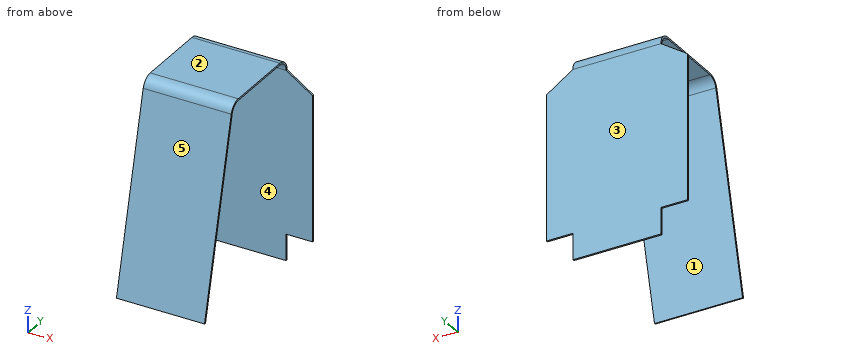
```python
from build123d import *

# Parameters (mm, degrees)
EXTRUDE_1_DEPTH      = 1.25
EXTRUDE_1_DEPTH_BACK = 1.25
SKETCH_2_W           = 4.631165465
SKETCH_2_H           = 0.05
EXTRUDE_1_2_DEPTH    = 0.75
CHAMFER_1_SIZE2      = 0.5
CHAMFER_1_SIZE       = 0.75
CHAMFER_2_SIZE2      = 0.5
CHAMFER_2_SIZE       = 0.75


with BuildPart() as part:
    # Эскиз1 → Extrude 1 (new, two sides: drawn at the far end of the back side and taken through both)
    with BuildSketch(Plane(origin=(0, 0, 0), x_dir=(0, 0, -1), z_dir=(1, 0, 0)).offset(-EXTRUDE_1_DEPTH_BACK)):
        with BuildLine():
            Line((0, 0), (-5.38, 0))
            ThreePointArc((-5.38, 0), (-5.592132034, -0.087867966), (-5.68, -0.3))
            Line((-5.68, -0.3), (-5.68, -2.314556047))
            ThreePointArc((-5.68, -2.314556047), (-5.615998777, -2.499770997), (-5.451302817, -2.60595939))
            Line((-5.451302817, -2.60595939), (-0.162763373, -3.9))
            Line((-0.162763373, -3.9), (-0.174647176, -3.948567224))
            Line((-0.174647176, -3.948567224), (-5.46318662, -2.654526614))
            ThreePointArc((-5.46318662, -2.654526614), (-5.655331906, -2.530640155), (-5.73, -2.314556047))
            Line((-5.73, -2.314556047), (-5.73, -0.3))
            ThreePointArc((-5.73, -0.3), (-5.627487373, -0.052512627), (-5.38, 0.05))
            Line((-5.38, 0.05), (0, 0.05))
            Line((0, 0.05), (0, 0))
        make_face()
    extrude(amount=EXTRUDE_1_DEPTH + EXTRUDE_1_DEPTH_BACK)

    # Эскиз2 → Extrude 1 2 (add)
    with BuildSketch(Plane(origin=(1.25, 0, 0), x_dir=(0, 0, -1), z_dir=(1, 0, 0))):
        with Locations((-3.064417268, 0.025)):
            Rectangle(SKETCH_2_W, SKETCH_2_H)
    extrude_1_2 = extrude(amount=EXTRUDE_1_2_DEPTH)

    # Фаска1
    chamfer_1_edges = [part.edges().sort_by_distance(p)[0] for p in [
        (2, 0.025, 5.38),
    ]]
    chamfer_1_side = [part.faces().sort_by_distance(p)[0] for p in [
        (1.99, 0.025, 5.38),
    ]]
    chamfer(chamfer_1_edges, length=CHAMFER_1_SIZE - 0.0001, length2=CHAMFER_1_SIZE2 - 0.0001, reference=chamfer_1_side[0])  # a hair under: the kernel refuses the full size

    # Зеркальное отражение1: Extrude 1 2 across plane
    add(extrude_1_2.mirror(Plane(origin=(0, 0, 0), x_dir=(0, 0, 1), z_dir=(1, 0, 0))))

    # Фаска2
    chamfer_2_edges = [part.edges().sort_by_distance(p)[0] for p in [
        (-2, 0.025, 5.38),
    ]]
    chamfer_2_side = [part.faces().sort_by_distance(p)[0] for p in [
        (-1.99, 0.025, 5.38),
    ]]
    chamfer(chamfer_2_edges, length=CHAMFER_2_SIZE - 0.0001, length2=CHAMFER_2_SIZE2 - 0.0001, reference=chamfer_2_side[0])  # a hair under: the kernel refuses the full size


solid = part.part
```
Could you check a few things on this model? Use its own coordinates, in mm. Face numbers are marked on the shaded views. A direction names the side the tool comes from. Round coordinates to 2 decimals unless told otherwise and drop trailing zeros. Loops run counter-clockwise (first coordinate to the right, second up) from the corner with the lowest first, then second, coordinate; pieces in that order, holes last. Notation, with made-up numbers: (14.25, 25.5) -> (21.25, 25.5) arc R5 cw to (21.25, 34.5) -> close; hole circle Ø6 at (40.25, -1.5). An arc over 180 degrees is marked (long way). Put each result on its own line as item: value.
Q1. I want a section at B-B on x = 0.85. Write out the boundary of the cut face in (y, z), and give its area (3 significant figures).
Checks:
outline: (-3.95, 0.17) -> (-3.9, 0.16) -> (-2.61, 5.45) arc R0.3 cw to (-2.31, 5.68) -> (-0.3, 5.68) arc R0.3 cw to (0, 5.38) -> (0, 0) -> (0.05, 0) -> (0.05, 5.38) arc R0.35 ccw to (-0.3, 5.73) -> (-2.31, 5.73) arc R0.35 ccw to (-2.65, 5.46) -> close
area: 0.689 mm2
Q2. I want a section at D-D on y = -2.5. Write out the boundary of the cut face in (x, z).
Checks:
outline: (-1.25, 5.62) -> (1.25, 5.62) -> (1.25, 5.68) -> (-1.25, 5.68) -> close
Q3. Which directions (+Z, -Z, +X, -X, +Y, -Y) give clear straight access to the entire face, cutting with the end or side of a thin tool? Please do the marked faces 1 and 2.
Checks:
face 1: -Z, +X, -X
face 2: +Z, +X, -X, +Y, -Y
Q4. Thinking about a two-plate mould opening in Y: for the marked faces 3, 4 and 5, which applies, pulls with the +Y half, pulls with the -Y half, needs draft (parallel to the pull), parting line crosses it, or undercut?
Checks:
face 3: pulls with the +Y half
face 4: undercut
face 5: pulls with the -Y half
Q5. I want a section at A-A on z = 1.2. Write out the boundary of the cut face in (x, y), and give its area (3 significant figures).
Checks:
outline: (-2, 0) -> (2, 0) -> (2, 0.05) -> (-2, 0.05) -> close; (-1.25, -3.7) -> (1.25, -3.7) -> (1.25, -3.65) -> (-1.25, -3.65) -> close
area: 0.329 mm2
Q6. For pin 1 Ø2 at (x, z) = (0.5, 2) entering from -Y; pin 2 Ø2 at (x, y) = (-1.5, -1.5) entering from -Z; pin 3 Ø1.2 at (y, z) = (-2.5, 3.5) entering from +X, each with a flat end and sliding along its axis, tell me the tip position at first contact or that it passes through.
Checks:
pin 1: y = -3.75
pin 2: z = 5.64
pin 3: x = 1.25
Q7. I want a section at C-C on y = -1.2. Write out the boundary of the cut face in (x, z), and give its area (3 significant figures).
Checks:
outline: (-1.25, 5.68) -> (1.25, 5.68) -> (1.25, 5.73) -> (-1.25, 5.73) -> close
area: 0.125 mm2
